Source: CAD feature listing. Evaluate the final solid. Frame: model axes, mm. Give positions to 0.01 mm unless a question says otherwise; leave off trailing zeros. Order: outer loops, then holes, each group sorted by start corner. A loop starts at its lowest first (then second) coordinate and runs counter-clockwise, first axis right, second up. Notation, with made-up numbers: (13.5, -24) - (71.5, -24) arc R26 cw to (71.5, -9) - close; hole circle Ø9 at (11, 17.5). An arc over 180 degrees is marked (long way). Write each question's results on one line, items separated by ' | '. Start each with the question number.
Item 1: Contact query for flat-ended pins moving along their axis: pin 1 Ø2 at (x, z) = (4.5, 80.5) entering from +Y; pin 2 Ø2 at (x, z) = (-5, 119) entering from +Y; pin 3 Ø2 at (y, z) = (-8.5, 71.5) entering from -X. Output: stop coordinate, or through.
Item 2: Section B-B on z = 23. Output: boundary loops of the cut face in (x, y).
Item 3: Line query: line 1 along X through (y, z) = (0, 67.5); line 2 along Y through (x, z) = (4, 46). Output: solid intervals per line, ascending.
Item 4: Mould query, pull axis X, two halves, no side actions, for faces 1 (the flat face through (-3.74, -8.03, -5.98)), 2 (the cylindrical face through (-1.389, -10.577, 73.148)), 3 (the flat face through (-6.7, 2.37, 145.17)), 4 (the cylindrical face through (-0.903, -6.875, 73.184)). Classes: released by +X, released by -X, zero draft, split by the parting line, or undercut.
Item 5: Section A-A on y = 4. Output: boundary loops of the cut face in (x, z), and give its area (3 significant figures).
Autodesk Inventor part; units mm, degrees
ref_plane "Start Plane" through (0, 0, -7.3433) normal (0, 0, 1) x (1, 0, 0)
ref_plane "End Plane" through (0, 0, 155.9241) normal (0, 0, 1) x (1, 0, 0)
ref_plane "Work Plane4" through (-9.359, -5.1201, 158.779) normal (0.6062, 0.3316, 0.7228) x (0.7867, -0.1167, -0.6062)
ref_plane "Start Plane" through (0, 0, -7.3433) normal (0, 0, 1) x (1, 0, 0)
ref_plane "End Plane" through (0, 0, 155.9241) normal (0, 0, 1) x (1, 0, 0)
sketch "Sketch" plane through (0, 0, 0) normal (0, 0, 1) x (1, 0, 0)
  circle A0 centre (0, 0) radius 6.9342
  circle A1 centre (0, 0) radius 10.668
  dimension "d0" = 21.336
  dimension "d1" = 3.7338
extrude "Body" add sketch "Sketch" along normal up to surface (163.2675 mm away) from surface at -7.3433
sketch "Sketch3" plane through (0, 0, 0) normal (0, 0, 1) x (1, 0, 0)
  line L0 (0, 0) -> (10, 0)
ref_plane "Work Plane3" through (0, 0, 0) normal (0, -1, 0) x (1, 0, 0)
sketch "Sketch4" plane through (0, 0, 0) normal (0, -1, 0) x (1, 0, 0)
  line L0 (-2, -7.3433) -> (12, -7.3433)
  line L1 (-2, 155.9241) -> (12, 155.9241)
  dimension "d7" = 163.2675
ref_plane "Work Plane4" through (-9.359, -5.1201, 158.779) normal (0.6062, 0.3316, 0.7228) x (0.7867, -0.1167, -0.6062)
split "Split1" plane through (-9.359, -5.1201, 158.779) removes the side toward (0.6062, 0.3316, 0.7228)
ref_plane "Work Plane5" through (-2.3452, -10.407, 155.9487) normal (0.1249, 0.5544, 0.8228) x (0.9914, -0.038, -0.1249)
split "Split2" plane through (-2.3452, -10.407, 155.9487) removes the side toward (0.1249, 0.5544, 0.8228)
ref_plane "Work Plane6" through (2.3628, -10.403, 158.1791) normal (-0.1481, 0.6522, 0.7434) x (0.9874, 0.0554, 0.1481)
split "Split3" plane through (2.3628, -10.403, 158.1791) removes the side toward (-0.1481, 0.6522, 0.7434)
ref_plane "Work Plane7" through (-9.359, -5.12, -10.1982) normal (0.6062, 0.3316, -0.7228) x (-0.326, -0.7254, -0.6062)
split "Split4" plane through (-9.359, -5.12, -10.1982) removes the side toward (0.6062, 0.3316, -0.7228)
ref_plane "Work Plane8" through (-2.3452, -10.407, -7.3679) normal (0.1249, 0.5544, -0.8228) x (0.9119, -0.3909, -0.1249)
split "Split5" plane through (-2.3452, -10.407, -7.3679) removes the side toward (0.1249, 0.5544, -0.8228)
ref_plane "Work Plane9" through (2.3628, -10.403, -9.5983) normal (-0.1481, 0.6522, -0.7434) x (0.9145, 0.3765, 0.1481)
split "Split6" plane through (2.3628, -10.403, -9.5983) removes the side toward (-0.1481, 0.6522, -0.7434)
equation "\"d0\" = G_H"
equation "\"d1\" = G_T"
equation "\"d2\" = G_L"
equation "\"G_H\" = 21.336"
equation "\"G_T\" = 3.7338"
equation "\"G_L\" = 163.26749"
equation "\"G_OFFSET_START\" = 7.34335"
equation "\"G_OFFSET_END\" = 7.34335"
equation "\"d4\" = -G_OFFSET_START"
equation "\"d5\" = G_OFFSET_END + B_L"
equation "\"B_L\" = 148.5808"
properties part number "ANSI - 1/2 x 0.147 - 6.428" material "Steel, Mild"
Evaluation:
1) pin 1: stops at y = 10.08 | pin 2: stops at y = 9.89 | pin 3: stops at x = -7.59
2) outline: circle Ø21.34 at (0, 0); hole circle Ø13.87 at (0, 0)
3) line 1: x = -10.67 to -6.93, 6.93 to 10.67 | line 2: y = -9.89 to -5.66, 5.66 to 9.89
4) face 1: released by +X | face 2: split by the parting line | face 3: released by -X | face 4: undercut
5) outline: (-9.89, 5.48) - (-5.66, 4.64) - (-5.66, 143.94) - (-9.89, 143.1) - close; (5.66, 6.59) - (9.89, 10.13) - (9.89, 138.45) - (5.66, 142) - close | area: 1,140 mm^2
